Build history of the part. All positions in model axes, mm. A direction names the side the tool comes from. Give positions to 0.01 mm unless a question says otherwise; leave off trailing zeros. Loops run counter-clockwise (first coordinate to the right, second up) from the corner with the lowest first, then second, coordinate; pieces in that order, holes last. Notation, with made-up numbers: M 27.5,53 L 52.5,53 A24 ccw 52.5,72 Z; hole C 60,-33.5 d4. An arc over 180 degrees is marked long. Answer in a Markdown table with one row per item. Add a question column.
```python
from build123d import *

# Parameters (mm, degrees)
SKETCH1_R           = 2
SKETCH1_W           = 40
SKETCH1_H           = 20
BOSS_EXTRUDE1_DEPTH = 10.7
SKETCH1_4_W         = 39
SKETCH1_4_H         = 30
BOSS_EXTRUDE2_DEPTH = 19
FILLET1_R           = 5
CUT_EXTRUDE2_REACH  = 21
SKETCH2_R           = 2.5


with BuildPart() as part:
    # Sketch1 → Boss-Extrude1 (new body)
    with BuildSketch(Plane(origin=(0, 0, 0), x_dir=(1, 0, 0), z_dir=(0, 1, 0))):
        Polygon((28, 15), (0, 15), (-28, 15), (-28, 0), (-28, -15), (0, -15), (33, -15), (33, 15), align=None)
        with Locations((-24.75, -5)):
            Circle(SKETCH1_R, mode=Mode.SUBTRACT)
        Rectangle(SKETCH1_W, SKETCH1_H, mode=Mode.SUBTRACT)
        with Locations((24.75, -5)):
            Circle(SKETCH1_R, mode=Mode.SUBTRACT)
        with Locations((-24.75, 5)):
            Circle(SKETCH1_R, mode=Mode.SUBTRACT)
        with Locations((24.75, 5)):
            Circle(SKETCH1_R, mode=Mode.SUBTRACT)
    extrude(amount=BOSS_EXTRUDE1_DEPTH)

    # Sketch1<4> → Boss-Extrude2 (add)
    with BuildSketch(Plane(origin=(0, 0, 0), x_dir=(1, 0, 0), z_dir=(0, 1, 0))):
        with Locations((52.5, 0)):
            Rectangle(SKETCH1_4_W, SKETCH1_4_H)
    extrude(amount=BOSS_EXTRUDE2_DEPTH)

    # Fillet1
    fillet1_edges = [part.edges().sort_by_distance(p)[0] for p in [
        (33, 10.7, 0),
    ]]
    fillet(fillet1_edges, radius=FILLET1_R)

    # Sketch2 → Cut-Extrude2 (cut, up to next)
    with BuildSketch(Plane.XZ, mode=Mode.PRIVATE) as cut_extrude2_sk1:
        with Locations((52.25, 0)):
            Circle(SKETCH2_R)
    cut_extrude2_tool1 = extrude(cut_extrude2_sk1.sketch, amount=-CUT_EXTRUDE2_REACH, mode=Mode.PRIVATE) & part.part
    add(cut_extrude2_tool1.solids().sort_by_distance((52.25, 0, 0))[0], mode=Mode.SUBTRACT)
    # Sketch2 → Cut-Extrude2 (cut, up to next)
    with BuildSketch(Plane.XZ, mode=Mode.PRIVATE) as cut_extrude2_sk2:
        with Locations((39.75, 10)):
            Circle(SKETCH2_R)
    cut_extrude2_tool2 = extrude(cut_extrude2_sk2.sketch, amount=-CUT_EXTRUDE2_REACH, mode=Mode.PRIVATE) & part.part
    add(cut_extrude2_tool2.solids().sort_by_distance((39.75, 0, 10))[0], mode=Mode.SUBTRACT)
    # Sketch2 → Cut-Extrude2 (cut, up to next)
    with BuildSketch(Plane.XZ, mode=Mode.PRIVATE) as cut_extrude2_sk3:
        with Locations((39.75, -10)):
            Circle(SKETCH2_R)
    cut_extrude2_tool3 = extrude(cut_extrude2_sk3.sketch, amount=-CUT_EXTRUDE2_REACH, mode=Mode.PRIVATE) & part.part
    add(cut_extrude2_tool3.solids().sort_by_distance((39.75, 0, -10))[0], mode=Mode.SUBTRACT)
    # Sketch2 → Cut-Extrude2 (cut, up to next)
    with BuildSketch(Plane.XZ, mode=Mode.PRIVATE) as cut_extrude2_sk4:
        with Locations((64.75, -10)):
            Circle(SKETCH2_R)
    cut_extrude2_tool4 = extrude(cut_extrude2_sk4.sketch, amount=-CUT_EXTRUDE2_REACH, mode=Mode.PRIVATE) & part.part
    add(cut_extrude2_tool4.solids().sort_by_distance((64.75, 0, -10))[0], mode=Mode.SUBTRACT)
    # Sketch2 → Cut-Extrude2 (cut, up to next)
    with BuildSketch(Plane.XZ, mode=Mode.PRIVATE) as cut_extrude2_sk5:
        with Locations((64.75, 10)):
            Circle(SKETCH2_R)
    cut_extrude2_tool5 = extrude(cut_extrude2_sk5.sketch, amount=-CUT_EXTRUDE2_REACH, mode=Mode.PRIVATE) & part.part
    add(cut_extrude2_tool5.solids().sort_by_distance((64.75, 0, 10))[0], mode=Mode.SUBTRACT)


solid = part.part
```
(1) Slice it at A-A, the plane x = 52.25. Give the cut face in (y, z).
(2) Slice it at B-B, the plane z = 0. Give the cut face in (x, y).
(3) Slice it at D-D, the plane y = 17.75. Give the cut face in (x, z), then the cut area to 3 significant figures.
(4) Tool access for faces 1 (the flat face through (0, 5, 10)), 2 (the flat face through (21, 0, 0)): list every direction of +Z, -Z, +X, -X, +Y, -Y with a clear straight run to the whole face (end or side of a thin tool).
(5) Pin check, flat tips, straight feed: pin 1 (8 mm diameter, centred on y = 15.5, z = 0.5, fed in from -X); pin 2 (15 mm diameter, centred on x = 10, z = -7, fed in from +Y); pin 3 (2.5 mm diameter, centred on y = 18, z = 2, fed in from -X). Stop position of each tip, or through.
(6) Pull direction Z, two halves, no side cores. Call faces 3 (the flat face through (32, 7, -15)), 4 (the cylindrical face through (42.06, 9.37, 9.04)), 5 (the flat face through (33, 17, 0)), 6 (the cylindrical face through (22.752, 5.275, -5.088)): +Z half, -Z half, draft (parallel to the pull), parting line (faces both ways), or undercut.
(7) Wall check: line 1 (X direction, y = 2.5, z = 5); line 2 (Z direction, x = -24.75, y = 4); line 3 (Z direction, x = 39.75, y = 10). Give the ranges that are in metal, low to high.
(8) Slice it at C-C, the plane y = 3. State how many separate pieces and enclosed holes the cut face has, then the cut area to 3 significant figures.
Solution:
| question | item | result |
|---|---|---|
| 1 | outline | M 0,-15 L 19,-15 L 19,-2.5 L 0,-2.5 Z; M 0,2.5 L 19,2.5 L 19,15 L 0,15 Z |
| 2 | outline | M -28,0 L -20,0 L -20,10.7 L -28,10.7 Z; M 20,0 L 49.75,0 L 49.75,19 L 33,19 L 33,15.7 A5 cw 28,10.7 L 20,10.7 Z; M 54.75,0 L 72,0 L 72,19 L 54.75,19 Z |
| 3 | outline | M 33,-15 L 72,-15 L 72,15 L 33,15 Z; hole C 39.75,-10 d5; hole C 39.75,10 d5; hole C 52.25,0 d5; hole C 64.75,-10 d5; hole C 64.75,10 d5 |
| 3 | area | 1,070 mm^2 |
| 4 | face 1 | +Y, -Y |
| 4 | face 2 | +Z, -Z, +X, -X, -Y |
| 5 | pin 1 | x = 30.71 |
| 5 | pin 2 | y = 10.7 |
| 5 | pin 3 | x = 33 |
| 6 | face 3 | -Z half |
| 6 | face 4 | undercut |
| 6 | face 5 | draft |
| 6 | face 6 | undercut |
| 7 | line 1 | -28 to -26.75, -22.75 to -20, 20 to 22.75, 26.75 to 72 |
| 7 | line 2 | -15 to -7, -3 to 3, 7 to 15 |
| 7 | line 3 | -15 to -12.5, -7.5 to 7.5, 12.5 to 15 |
| 8 | separate pieces | 1 |
| 8 | enclosed holes | 10 |
| 8 | area | 2,050 mm^2 |
